from build123d import *

# Parameters (mm, degrees)
SKETCH_2_W          = 46
SKETCH_2_H          = 46
EXTRUDE_1_DEPTH     = 10
SKETCH_4_R          = 55
SKETCH_4_R_2        = 1.6
EXTRUDE_2_DEPTH     = 10
SKETCH_5_R          = 55
EXTRUDE_3_DEPTH     = 10
SKETCH_6_R          = 1.5
SKETCH_6_W          = 5
SKETCH_6_H          = 30
CUT_EXTRUDE_1_DEPTH = 320.501564941
FILLET_1_R          = 20


with BuildPart() as part:
    # 草图2 → 凸台-拉伸1 (new body)
    with BuildSketch(Plane(origin=(0, 0, 0), x_dir=(1, 0, 0), z_dir=(0, 1, 0))):
        Rectangle(SKETCH_2_W, SKETCH_2_H)
    extrude(amount=EXTRUDE_1_DEPTH)

    # 草图4 → 凸台-拉伸2 (add)
    with BuildSketch(Plane(origin=(0, 10, 0), x_dir=(1, 0, 0), z_dir=(0, 1, 0))):
        with Locations(Location((0, 0, 0), (0, 0, 270))):
            Circle(SKETCH_4_R)
        with Locations(Location((-49.1, 0, 0), (0, 0, 270))):
            Circle(SKETCH_4_R_2, mode=Mode.SUBTRACT)
        with Locations(Location((0, -49.1, 0), (0, 0, 270))):
            Circle(SKETCH_4_R_2, mode=Mode.SUBTRACT)
        with Locations(Location((49.1, 0, 0), (0, 0, 270))):
            Circle(SKETCH_4_R_2, mode=Mode.SUBTRACT)
        with Locations(Location((0, 49.1, 0), (0, 0, 270))):
            Circle(SKETCH_4_R_2, mode=Mode.SUBTRACT)
    extrude(amount=-EXTRUDE_2_DEPTH)

    # 草图5 → 凸台-拉伸3 (add)
    with BuildSketch(Plane(origin=(0, 10, 0), x_dir=(1, 0, 0), z_dir=(0, 1, 0))):
        Polygon((30, -233.826859022), (30, -51.961524227), (187.5, -142.894191624), (217.5, -90.932667397), (60, 0), (217.5, 90.932667397), (187.5, 142.894191624), (30, 51.961524227), (30, 233.826859022), (-30, 233.826859022), (-30, 51.961524227), (-187.5, 142.894191624), (-217.5, 90.932667397), (-60, 0), (-217.5, -90.932667397), (-187.5, -142.894191624), (-30, -51.961524227), (-30, -233.826859022), align=None)
        Circle(SKETCH_5_R, mode=Mode.SUBTRACT)
    extrude(amount=-EXTRUDE_3_DEPTH)

    # 草图6 → 切除-拉伸1 (cut, through all)
    with BuildSketch(Plane(origin=(0, 10, 0), x_dir=(1, 0, 0), z_dir=(0, 1, 0))):
        with Locations(Location((0, 218.826859022, 0), (0, 0, 270))):
            Circle(SKETCH_6_R)
        with Locations(Location((189.509618943, 109.413429511, 0), (0, 0, 270))):
            Circle(SKETCH_6_R)
        with Locations(Location((189.509618943, -109.413429511, 0), (0, 0, 270))):
            Circle(SKETCH_6_R)
        with Locations(Location((0, -218.826859022, 0), (0, 0, 270))):
            Circle(SKETCH_6_R)
        with Locations(Location((-189.509618943, -109.413429511, 0), (0, 0, 270))):
            Circle(SKETCH_6_R)
        with Locations(Location((-189.509618943, 109.413429511, 0), (0, 0, 270))):
            Circle(SKETCH_6_R)
        Polygon((152.804445662, 85.334936491), (150.304445662, 89.665063509), (176.285207776, 104.665063509), (178.785207776, 100.334936491), align=None)
        with Locations((0, 190)):
            Rectangle(SKETCH_6_W, SKETCH_6_H)
        with Locations((0, 110)):
            Rectangle(SKETCH_6_W, SKETCH_6_H)
        Polygon((83.52241336, 45.334936491), (81.02241336, 49.665063509), (107.003175473, 64.665063509), (109.503175473, 60.334936491), align=None)
        Polygon((-107.003175473, -64.665063509), (-109.503175473, -60.334936491), (-83.52241336, -45.334936491), (-81.02241336, -49.665063509), align=None)
        Polygon((81.02241336, -49.665063509), (83.52241336, -45.334936491), (109.503175473, -60.334936491), (107.003175473, -64.665063509), align=None)
        Polygon((-109.503175473, 60.334936491), (-107.003175473, 64.665063509), (-81.02241336, 49.665063509), (-83.52241336, 45.334936491), align=None)
        Polygon((-176.285207776, -104.665063509), (-178.785207776, -100.334936491), (-152.804445662, -85.334936491), (-150.304445662, -89.665063509), align=None)
        Polygon((150.304445662, -89.665063509), (152.804445662, -85.334936491), (178.785207776, -100.334936491), (176.285207776, -104.665063509), align=None)
        Polygon((-178.785207776, 100.334936491), (-176.285207776, 104.665063509), (-150.304445662, 89.665063509), (-152.804445662, 85.334936491), align=None)
        with Locations((0, -110)):
            Rectangle(SKETCH_6_W, SKETCH_6_H)
        with Locations((0, -190)):
            Rectangle(SKETCH_6_W, SKETCH_6_H)
    extrude(amount=-CUT_EXTRUDE_1_DEPTH, mode=Mode.SUBTRACT)

    # 圆角1
    fillet_1_edges = [part.edges().sort_by_distance(p)[0] for p in [
        (187.5, 5, -142.894191624),
        (217.5, 5, -90.932667397),
        (60, 5, 0),
        (217.5, 5, 90.932667397),
        (187.5, 5, 142.894191624),
        (30, 5, 51.961524227),
        (30, 5, 233.826859022),
        (-30, 5, 233.826859022),
        (-30, 5, 51.961524227),
        (-187.5, 5, 142.894191624),
        (-217.5, 5, 90.932667397),
        (-60, 5, 0),
        (-217.5, 5, -90.932667397),
        (-187.5, 5, -142.894191624),
        (-30, 5, -51.961524227),
        (-30, 5, -233.826859022),
        (30, 5, -233.826859022),
        (30, 5, -51.961524227),
    ]]
    fillet(fillet_1_edges, radius=FILLET_1_R)


solid = part.part
Model file for the job. Use its own axes, mm. A direction names the side the tool comes from. Give positions to 0.01 mm unless a question says otherwise; leave off trailing zeros. Order: outer loops, then holes, each group sorted by start corner. A loop starts at its lowest first (then second) coordinate and runs counter-clockwise, first axis right, second up. Notation, with made-up numbers: (89, 88) -> (115, 88) arc R7 cw to (115, 99) -> close; hole circle Ø3 at (70, 48). An arc over 180 degrees is marked (long way). Use CSV: the item, a comma, the result in double quotes.
1. Band-saw the part on B-B, the plane x = -117. Give the cut face in (y, z), then the cut area to 3 significant figures.
Outcome:
outline,"(0, -102.19) -> (10, -102.19) -> (10, -32.91) -> (0, -32.91) -> close; (0, 32.91) -> (10, 32.91) -> (10, 102.19) -> (0, 102.19) -> close"
area,"1,390 mm²"
2. Band-saw the part on D-D, the plane x = 67. Give the cut face in (y, z).
Outcome:
outline,"(0, -73.32) -> (10, -73.32) -> (10, 73.32) -> (0, 73.32) -> close"
3. Mould opens along Z. For faces 4 (the flat face through (2.5, 5, -110)), 5 (the flat face through (30, 5, 151)), 6 (the flat face through (-115.861, 5.07, 101.533)) say: +Z half, -Z half, draft (parallel to the pull), parting line (faces both ways), or undercut.
Outcome:
face 4,"undercut"
face 5,"draft"
face 6,"+Z half"
4. Band-saw the part on A-A, the plane z = 192.5. Give the cut face in (x, y).
Outcome:
outline,"(-30, 0) -> (-2.5, 0) -> (-2.5, 10) -> (-30, 10) -> close; (2.5, 0) -> (30, 0) -> (30, 10) -> (2.5, 10) -> close"
5. Drill centre lines: line 1 along X through (y, z) = (4.5, 0); line 2 along Z through (x, y) = (-155, 0.5); line 3 along X through (y, z) = (7.5, -81). Where is each one in solid material? Low to high. Write a range as from..to.
Outcome:
line 1,"-80..-50.7, -47.5..47.5, 50.7..80"
line 2,"-124.13..-92.38, -86.6..-54.85, 54.85..86.6, 92.38..124.13"
line 3,"-200.3..-80.3, -30.8..30.8, 80.3..200.3"
6. Band-saw the part on C-C, the plane y = 7.5. Count the separate pieces of the cut face and the enclosed holes in it, then the cut area to 3 significant figures.
Outcome:
separate pieces,"1"
enclosed holes,"22"
area,"73,600 mm²"
7. Drop flat-ended pins along their axis: pin 1 (2.5 mm diameter, centred on x = 0, z = 218.83, fed in from +Y); pin 2 (5 mm diameter, centred on x = -103.5, y = 4.5, fed in from +Z); pin 3 (5 mm diameter, centred on y = 8, z = 49.5, fed in from +X); pin 4 (6 mm diameter, centred on x = 46.5, y = 6.5, fed in from +Z). Give the stop position or say it passes through.
Outcome:
pin 1,"through"
pin 2,"z = 95.84"
pin 3,"x = 150.07"
pin 4,"z = 67.69"
8. 3-axis set-ups, long thin cutter, end or side, ignore diameter. For faces 1 (the flat face through (165.98, 5.07, -92.94)), 2 (the flat face through (145.86, 5.07, 49.57)), 3 (the flat face through (30, 5, -149)): which of +Z, -Z, +X, -X, +Y, -Y reach the whole face in a straight line?
Outcome:
face 1,"+Y, -Y"
face 2,"+X, +Y, -Y"
face 3,"-Z, +Y, -Y"
